Work out the finished part from the listing and answer in its coordinate system (mm). A direction names the side the tool comes from. Round coordinates to 2 decimals unless told otherwise and drop trailing zeros. Write each loop counter-clockwise with the first axis right and the second up, starting at its lowest first coordinate (ties: lowest second). Pieces come first, ordered by that corner, then holes. Notation, with made-up numbers: (-1.75, 34.25) -> (51.25, 34.25) arc R27 ccw to (51.25, 56.25) -> close; hole circle Ø8 at (60, 50.25). An arc over 180 degrees is marked (long way). Answer as a JSON object with one key per item and string values. Group by question number.
from build123d import *

# Parameters (mm, degrees)
SKETCH2_R                 = 55
SKETCH2_W                 = 30
SKETCH2_H                 = 14
BOSS_EXTRUDE1_DEPTH       = 5
SKETCH3_R                 = 2.5
BOSS_EXTRUDE2_DEPTH       = 6
F_2_5MM_DOWEL_HOLE2_D     = 2.5
F_2_5MM_DOWEL_HOLE2_DEPTH = 10.15
F_2_5MM_DOWEL_HOLE2_TIP   = 0.751075774
SKETCH15_R                = 1.55
BOSS_EXTRUDE3_DEPTH       = 9.5
F_2_0MM_DOWEL_HOLE1_D     = 2
F_2_0MM_DOWEL_HOLE1_DEPTH = 10.15
F_2_0MM_DOWEL_HOLE1_TIP   = 0.600860619
SKETCH17_R                = 1.55
SKETCH17_W                = 14.2
SKETCH17_H                = 5
BOSS_EXTRUDE4_DEPTH       = 9.5
F_2_0MM_DOWEL_HOLE2_D     = 2
F_2_0MM_DOWEL_HOLE2_DEPTH = 10.15
F_2_0MM_DOWEL_HOLE2_TIP   = 0.600860619
SKETCH19_W                = 14.2
SKETCH19_H                = 5
BOSS_EXTRUDE5_DEPTH       = 4
SKETCH21_W                = 10
SKETCH21_H                = 10
CUT_EXTRUDE1_DEPTH        = 79.944600829
SKETCH26_R                = 3
BOSS_EXTRUDE7_DEPTH       = 3
F_3_0MM_DOWEL_HOLE2_D     = 3
SKETCH30_R                = 3
BOSS_EXTRUDE9_DEPTH       = 33
F_3_0MM_DOWEL_HOLE4_D     = 3


with BuildPart() as part:
    # Sketch2 → Boss-Extrude1 (new body)
    with BuildSketch(Plane(origin=(0, 0, 0), x_dir=(1, 0, 0), z_dir=(0, 1, 0))):
        with Locations(Location((0, 0, 0), (0, 0, 270))):
            Circle(SKETCH2_R)
        with Locations((0, -30)):
            Rectangle(SKETCH2_W, SKETCH2_H, mode=Mode.SUBTRACT)
    extrude(amount=BOSS_EXTRUDE1_DEPTH)

    # Sketch3 → Boss-Extrude2 (add)
    with BuildSketch(Plane.XZ):
        with Locations(Location((-36.95, 10.6, 0), (0, 0, 90))):
            Circle(SKETCH3_R)
        with Locations(Location((-36.95, -10.6, 0), (0, 0, 90))):
            Circle(SKETCH3_R)
        with Locations(Location((6.95, -10.6, 0), (0, 0, 90))):
            Circle(SKETCH3_R)
        with Locations(Location((6.95, 10.6, 0), (0, 0, 90))):
            Circle(SKETCH3_R)
    extrude(amount=BOSS_EXTRUDE2_DEPTH)

    # 2.5mm Dowel Hole2
    with Locations(Plane(origin=(-36.95, -6, 10.6), x_dir=(0, 0, -1), z_dir=(0, -1, 0))):
        with Locations((0, 0), (0, 43.9), (21.2, 43.9), (21.2, 0)):
            Hole(F_2_5MM_DOWEL_HOLE2_D / 2, depth=F_2_5MM_DOWEL_HOLE2_DEPTH)
            with Locations((0, 0, -(F_2_5MM_DOWEL_HOLE2_DEPTH + F_2_5MM_DOWEL_HOLE2_TIP / 2))):  # 118° drill point
                Cone(0, F_2_5MM_DOWEL_HOLE2_D / 2, F_2_5MM_DOWEL_HOLE2_TIP, mode=Mode.SUBTRACT)

    # Sketch15 → Boss-Extrude3 (add)
    with BuildSketch(Plane(origin=(0, 5, 0), x_dir=(1, 0, 0), z_dir=(0, 1, 0))):
        with Locations(Location((-30.02607336, 29.209873591, 0), (0, 0, 270))):
            Circle(SKETCH15_R)
        with Locations(Location((-14.37607336, 29.209873591, 0), (0, 0, 90))):
            Circle(SKETCH15_R)
        with Locations(Location((-14.37607336, 1.709873591, 0), (0, 0, 270))):
            Circle(SKETCH15_R)
        with Locations(Location((-30.02607336, 1.709873591, 0), (0, 0, 90))):
            Circle(SKETCH15_R)
    extrude(amount=BOSS_EXTRUDE3_DEPTH)

    # 2.0mm Dowel Hole1
    with Locations(Plane(origin=(-30.02607336, 14.5, -29.209873591), x_dir=(0, 0, 1), z_dir=(0, 1, 0))):
        with Locations((0, 0), (27.5, 0), (27.5, 15.65), (0, 15.65)):
            Hole(F_2_0MM_DOWEL_HOLE1_D / 2, depth=F_2_0MM_DOWEL_HOLE1_DEPTH)
            with Locations((0, 0, -(F_2_0MM_DOWEL_HOLE1_DEPTH + F_2_0MM_DOWEL_HOLE1_TIP / 2))):  # 118° drill point
                Cone(0, F_2_0MM_DOWEL_HOLE1_D / 2, F_2_0MM_DOWEL_HOLE1_TIP, mode=Mode.SUBTRACT)

    # Sketch17 → Boss-Extrude4 (add)
    with BuildSketch(Plane(origin=(0, 5, 0), x_dir=(1, 0, 0), z_dir=(0, 1, 0))):
        with Locations(Location((19.217395201, 5, 0), (0, 0, 270))):
            Circle(SKETCH17_R)
        with Locations((19.217395201, 30.5)):
            Rectangle(SKETCH17_W, SKETCH17_H)
    extrude(amount=BOSS_EXTRUDE4_DEPTH)

    # 2.0mm Dowel Hole2
    with Locations(Plane(origin=(19.217395201, 14.5, -5), x_dir=(0, 0, 1), z_dir=(0, 1, 0))):
        with Locations((0, 0)):
            Hole(F_2_0MM_DOWEL_HOLE2_D / 2, depth=F_2_0MM_DOWEL_HOLE2_DEPTH)
            with Locations((0, 0, -(F_2_0MM_DOWEL_HOLE2_DEPTH + F_2_0MM_DOWEL_HOLE2_TIP / 2))):  # 118° drill point
                Cone(0, F_2_0MM_DOWEL_HOLE2_D / 2, F_2_0MM_DOWEL_HOLE2_TIP, mode=Mode.SUBTRACT)

    # Sketch19 → Boss-Extrude5 (add)
    with BuildSketch(Plane(origin=(0, 14.5, 0), x_dir=(1, 0, 0), z_dir=(0, 1, 0))):
        with Locations((19.217395201, 30.5)):
            Rectangle(SKETCH19_W, SKETCH19_H)
    extrude(amount=BOSS_EXTRUDE5_DEPTH)

    # Sketch21 → Cut-Extrude1 (cut, through all)
    with BuildSketch(Plane(origin=(0, 5, 0), x_dir=(1, 0, 0), z_dir=(0, 1, 0))):
        with Locations((-50, 0)):
            Rectangle(SKETCH21_W, SKETCH21_H)
    extrude(amount=-CUT_EXTRUDE1_DEPTH, mode=Mode.SUBTRACT)

    # Sketch26 → Boss-Extrude7 (add)
    with BuildSketch(Plane.XZ):
        with Locations(Location((0, 42, 0), (0, 0, 90))):
            Circle(SKETCH26_R)
        with Locations(Location((0, -37, 0), (0, 0, 90))):
            Circle(SKETCH26_R)
    extrude(amount=BOSS_EXTRUDE7_DEPTH)

    # 3.0mm Dowel Hole2 (through all)
    with Locations(Plane(origin=(0, -3, 42), x_dir=(0, 0, -1), z_dir=(0, -1, 0))):
        with Locations((0, 0), (79, 0)):
            Hole(F_3_0MM_DOWEL_HOLE2_D / 2)

    # Sketch30 → Boss-Extrude9 (add)
    with BuildSketch(Plane.XZ):
        with Locations(Location((-36, 30, 0), (0, 0, 90))):
            Circle(SKETCH30_R)
        with Locations(Location((36, 30, 0), (0, 0, 90))):
            Circle(SKETCH30_R)
        with Locations(Location((36, -30, 0), (0, 0, 90))):
            Circle(SKETCH30_R)
        with Locations(Location((-36, -30, 0), (0, 0, 90))):
            Circle(SKETCH30_R)
    extrude(amount=BOSS_EXTRUDE9_DEPTH)

    # 3.0mm Dowel Hole4 (through all)
    with Locations(Plane(origin=(-36, -33, 30), x_dir=(0, 0, -1), z_dir=(0, -1, 0))):
        with Locations((0, 0), (0, 72), (60, 72), (60, 0)):
            Hole(F_3_0MM_DOWEL_HOLE4_D / 2)


solid = part.part
1) A cutting plane is placed at D-D on x = -6.5. Determine the outline of the cut face in (y, z), plus the area to 3 significant figures.
2) Each of these flat-tipped pins is pushed along its axis until it touches: P1, Ø1.2, axis at x = -14.38, z = -29.21, coming from the -Y side; P2, Ø6.5, axis at x = 0, z = -37, coming from the -Y side; P3, Ø2.5, axis at x = -14, z = -2, coming from the +Y side. Where does it stop, or does it pass through?
3) A tool of negligible diameter and unlimited length cuts with its end or side. For faces 1 (the face through (-36, -6, -12)), 2 (the face through (-50, 3, -5)), 3 (the face through (26.317, 12, -30)), from which of +Z, -Z, +X, -X, +Y, -Y can it reach the whole face along a straight path? Write none if from no direction.
4) A cutting plane is placed at B-B on y = -1.5. State how many separate pieces and enclosed holes the cut face has, plus the area to 3 significant figures.
5) A cutting plane is placed at A-A on y = -25. Determine the outline of the cut face in (x, z), plus the area to 3 significant figures.
6) For a pull along X with two mould halves and no side action, classify faces 4 (the face through (17.704, 9.683, -5.336)), 5 (the face through (-15, 2, 30)), 6 (the face through (1, 0, -1)), 7 (the face through (-34.7, -33, -28.7)) as released by +X, released by -X, zero draft, split by the parting line, or undercut.
7) Straight lines are drawn through the part: L1, parallel to Z at x = 37, y = -4.5; L2, parallel to X at y = -4, z = 31; L3, parallel to Y at x = 43, z = 6. For each, find the intervals that lie inside material, in ascending order.
8) A cutting plane is placed at C-C on z = 30. Determine the outline of the cut face in (x, y), plus the area to 3 significant figures.
Established:
{
 "1": {"outline": "(0, -54.61) -> (5, -54.61) -> (5, 23) -> (0, 23) -> close; (0, 37) -> (5, 37) -> (5, 54.61) -> (0, 54.61) -> close", "area": "476 mm²"},
 "2": {"P1": "stops at y = 0", "P2": "stops at y = -3", "P3": "stops at y = 14.5"},
 "3": {"face 1": "+X, -X, -Y", "face 2": "-X, +Y, -Y", "face 3": "+Z, -Z, +X, +Y"},
 "4": {"separate pieces": "10", "enclosed holes": "10", "area": "186 mm²"},
 "5": {"outline": "circle Ø6 at (-36, -30); circle Ø6 at (-36, 30); circle Ø6 at (36, -30); circle Ø6 at (36, 30); hole circle Ø3 at (-36, -30); hole circle Ø3 at (-36, 30); hole circle Ø3 at (36, -30); hole circle Ø3 at (36, 30)", "area": "84.8 mm²"},
 "6": {"face 4": "split by the parting line", "face 5": "undercut", "face 6": "undercut", "face 7": "zero draft"},
 "7": {"L1": "z = -32.83 to -31.12, -28.88 to -27.17, 27.17 to 28.88, 31.12 to 32.83", "L2": "x = -38.83 to -37.12, -34.88 to -33.17, 33.17 to 34.88, 37.12 to 38.83", "L3": "y = 0 to 5"},
 "8": {"outline": "(-46.1, 0) -> (-39, 0) -> (-39, -33) -> (-37.5, -33) -> (-37.5, 5) -> (-46.1, 5) -> close; (-34.5, -33) -> (-33, -33) -> (-33, 0) -> (-15, 0) -> (-15, 5) -> (-34.5, 5) -> close; (15, 0) -> (33, 0) -> (33, -33) -> (34.5, -33) -> (34.5, 5) -> (15, 5) -> close; (37.5, -33) -> (39, -33) -> (39, 0) -> (46.1, 0) -> (46.1, 5) -> (37.5, 5) -> close", "area": "479 mm²"}
}
